from build123d import *


with BuildPart() as f4:
    # F4: sweep along a path in F2
    with BuildLine(Plane.XY.offset(60)) as f4_path:
        Line((-46.337677, 0), (-46.337677, -58.146937))
        ThreePointArc((-46.337677, -58.146937), (-39.894026, -73.703286), (-24.337677, -80.146937))
        Line((-24.337677, -80.146937), (24.337677, -80.146937))
        ThreePointArc((24.337677, -80.146937), (39.894026, -73.703286), (46.337677, -58.146937))
        Line((46.337677, -58.146937), (46.337677, 0))
    # F3 (on Front) → F4 (sweep)
    with BuildSketch(Plane.XZ):
        with BuildLine():
            Line((-44.345288, 60.174311), (-46.337677, 60))
            Line((-46.337677, 60), (-41.676718, 6.724992))
            ThreePointArc((-41.676718, 6.724992), (-39.314801, 1.935497), (-34.337677, 0))
            Line((-34.337677, 0), (-34.337677, 2))
            ThreePointArc((-34.337677, 2), (-37.96362, 3.410052), (-39.684328, 6.899303))
            Line((-39.684328, 6.899303), (-44.345288, 60.174311))
        make_face()
    sweep(path=f4_path.line)


solid = f4.part
Here's how the part is built. I have some questions about the finished solid (model axes, mm). A direction names the side the tool comes from. Round coordinates to 2 decimals unless told otherwise and drop trailing zeros. Loops run counter-clockwise (first coordinate to the right, second up) from the corner with the lowest first, then second, coordinate; pieces in that order, holes last.
1. If we section it at A-A on z = 46: Write out the boundary of the cut face in (x, y).
Answer list:
outline: (-45.11, -58.15) arc R20.78 ccw to (-24.34, -78.92) - (24.34, -78.92) arc R20.78 ccw to (45.11, -58.15) - (45.11, 0) - (43.11, 0) - (43.11, -58.15) arc R18.77 cw to (24.34, -76.91) - (-24.34, -76.91) arc R18.77 cw to (-43.11, -58.15) - (-43.11, 0) - (-45.11, 0) - close
2. Which directions (+Z, -Z, +X, -X, +Y, -Y) give clear straight access to the entire face, cutting with the end or side of a thin tool? Please do faces 5 (the face through (0.34, -75.79, 33.16)), 6 (the face through (-38.375, -71.879, 32.99)), 7 (the face through (31.331, -65.295, 1.014)).
Answer list:
face 5: +Z, +Y
face 6: -Z, -X, -Y
face 7: +Z, -Z, +Y
3. We'd pull the mould along X, two halves only. Please class faces 1 (the face through (44.04, -28.67, 33.74)), 2 (the face through (-38.887, -72.38, 60.144)), 3 (the face through (36.72, -70.81, 33.91)), 4 (the face through (-31.486, -65.14, 1.014)): +X half, -X half, draft (parallel to the pull), parting line (faces both ways), or undercut.
Answer list:
face 1: +X half
face 2: -X half
face 3: undercut
face 4: undercut
4. For P1, Ø12, axis at x = 6, z = 21, coming from the -Y side; P2, Ø12, axis at x = 31.5, y = -28, coming from the +Z side; P3, Ø1.5, axis at x = 19.5, z = 24, coming from the +Y side, each with a flat end and sliding along its axis, tell me the tip position at first contact or that it passes through.
Answer list:
P1: stops at y = -77.26
P2: stops at z = 3.03
P3: stops at y = -74.92
5. If I drill on line 1 along X through (y, z) = (-72.5, 26); line 2 along X through (y, z) = (-44, 46.5); line 3 along Y through (x, z) = (-2, 37.5), over which ranges is the centre line in solid material (lowest first)?
Answer list:
line 1: x = -36.83 to -33.48, 33.48 to 36.83
line 2: x = -45.16 to -43.15, 43.15 to 45.16
line 3: y = -78.18 to -76.17
6. If we section it at B-B on z = 13: Write out the boundary of the cut face in (x, y), plus the area to 3 significant figures.
Answer list:
outline: (-42.23, -58.15) arc R17.89 ccw to (-24.34, -76.03) - (24.34, -76.03) arc R17.89 ccw to (42.23, -58.15) - (42.23, 0) - (40.22, 0) - (40.22, -58.15) arc R15.88 cw to (24.34, -74.03) - (-24.34, -74.03) arc R15.88 cw to (-40.22, -58.15) - (-40.22, 0) - (-42.23, 0) - close
area: 438 mm2
